Study the drawing (mm; zero at the part's minimum x, y, z) and answer. A direction names the side the tool comes from. Round coordinates to 2 decimals unless told otherwise and drop trailing zeros. Order: outer loops, then holes, each group sorted by start corner. A loop starts at its lowest first (then second) coordinate and runs counter-clockwise, first axis right, second up. Notation, with made-up numbers: M 14.25,-12.5 L 49.25,-12.5 A5 cw 49.25,-6.5 Z; hole C 89,46 d5. An arc over 180 degrees is marked long. Put each result on its own line as item: value. Start each with the question number.
1. Consider line 1 (Z direction, x = 3.5, y = 20.25); line 2 (Y direction, x = 13, z = 50.5); line 3 (X direction, y = 14, z = 108). Determine where each line is inside the solid, lowest interval first.
2. The part is cut by section C-C (z = 34). Give the vertices of the cut face in (x, y).
3. The mould has two halves that part along Z. Classify the marked faces 3, 4 and 5: +Z half, -Z half, draft (parallel to the pull), parting line (faces both ways), or undercut.
4. Each of these flat-tipped pins is pushed along its axis until it touches: pin 1 Ø6 at (x, z) = (17, 94.5) entering from +Y; pin 2 Ø8 at (x, z) = (20, 15.5) entering from -Y; pin 3 Ø2 at (y, z) = (9, 30.5) entering from +X. Where does it stop, or does it pass through?
5. The part is cut by section B-B (x = 4). Give the vertices of the cut face in (y, z), then the cut area to 3 significant figures.
6. The part is cut by section A-A (y = 24.25). Give the vertices of the cut face in (x, z), then the cut area to 3 significant figures.
7. Which of the six approach directions +Z, -Z, +X, -X, +Y, -Y give full straight-line access (tool end or side, diameter ignored) to the marked faces 1 and 2?
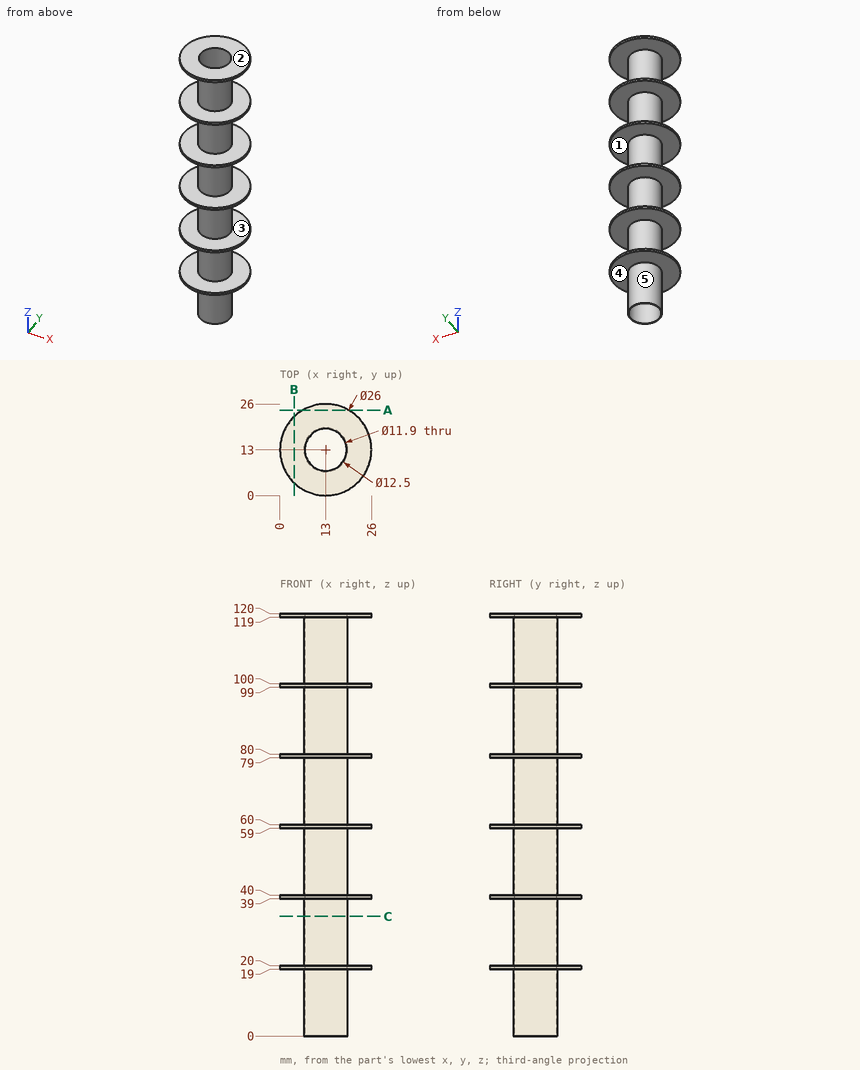
Resolved:
1. line 1: 19 to 20, 39 to 40, 59 to 60, 79 to 80, 99 to 100, 119 to 120
1. line 2: 6.75 to 7.05, 18.95 to 19.25
1. line 3: 6.83 to 7.13, 18.87 to 19.17
2. outline: C 13,13 d12.5; hole C 13,13 d11.9
3. face 3: undercut
3. face 4: -Z half
3. face 5: draft
4. pin 1: y = 19.17
4. pin 2: y = 1.03
4. pin 3: x = 18.48
5. outline: M 3.62,19 L 22.38,19 L 22.38,20 L 3.62,20 Z; M 3.62,39 L 22.38,39 L 22.38,40 L 3.62,40 Z; M 3.62,59 L 22.38,59 L 22.38,60 L 3.62,60 Z; M 3.62,79 L 22.38,79 L 22.38,80 L 3.62,80 Z; M 3.62,99 L 22.38,99 L 22.38,100 L 3.62,100 Z; M 3.62,119 L 22.38,119 L 22.38,120 L 3.62,120 Z
5. area: 113 mm2
6. outline: M 6.49,19 L 19.51,19 L 19.51,20 L 6.49,20 Z; M 6.49,39 L 19.51,39 L 19.51,40 L 6.49,40 Z; M 6.49,59 L 19.51,59 L 19.51,60 L 6.49,60 Z; M 6.49,79 L 19.51,79 L 19.51,80 L 6.49,80 Z; M 6.49,99 L 19.51,99 L 19.51,100 L 6.49,100 Z; M 6.49,119 L 19.51,119 L 19.51,120 L 6.49,120 Z
6. area: 78.2 mm2
7. face 1: none
7. face 2: +Z, +X, -X, +Y, -Y
